Verification items for the finished model (mm, model axes). Face numbers are marked on the shaded views. A direction names the side the tool comes from. Give positions to 0.01 mm unless a question says otherwise; leave off trailing zeros. Write each loop counter-clockwise with the first axis right and the second up, starting at its lowest first coordinate (ties: lowest second). Pieces come first, ordered by that corner, then holes. Notation, with made-up numbers: (73, 13) -> (84, 13) arc R12 cw to (84, 23) -> close; hole circle Ø3 at (12, 29). An arc over 180 degrees is marked (long way). Use one line per item in the form item = value. Start each with the question number.
(1) Set-up check for the marked faces 1 and 2: record each of +Z, -Z, +X, -X, +Y, -Y from which the full face is reachable in a straight line by a thin tool's end or side.
(2) Section check D-D, the plane x = 39.5. Record the cut outline in (y, z).
(3) Scan lines: L1, parallel to X at y = 3.9, z = 0; L2, parallel to Z at x = -62.5, y = 6; L3, parallel to Z at x = 22, y = 15. Record each from-to range of solid material in increasing order.
(4) Section check B-B, the plane x = -38.5. Record the cut outline in (y, z), plus the area to 3 significant figures.
(5) Release check for a two-part mould opening along Z. For the marked faces 3, 4, 5 and 6 record: pulls with the +Z half, pulls with the -Z half, needs draft (parallel to the pull), parting line crosses it, or undercut.
(6) Depth check by flat-ended pin: pin 1 Ø5 at (x, z) = (-31, 19.5) entering from +Y; pin 2 Ø8 at (x, z) = (39.5, -0.5) entering from +Y; pin 3 Ø10 at (y, z) = (13.5, 6.5) entering from -X. Enter the tip coordinate at first touch or a pass-through.
(7) Section check A-A, the plane y = 5. Record the cut outline in (x, z) (3 decimals).
(8) Section check C-C, the plane x = 55. Record the cut outline in (y, z), plus the area to 3 significant figures.
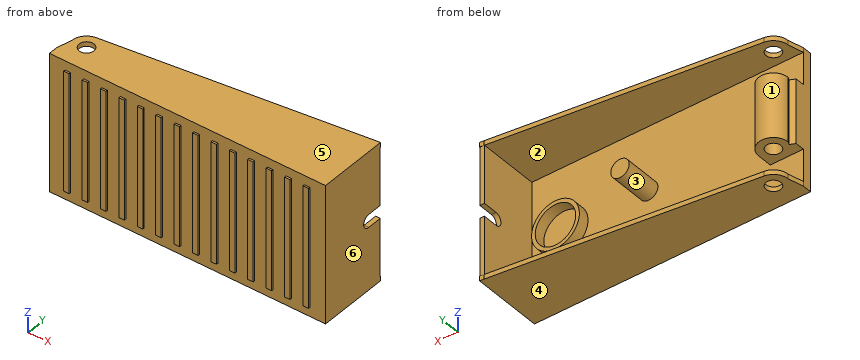
from build123d import *

# Parameters (mm, degrees)
SKETCH2_W               = 150
SKETCH2_H               = 75
BOSS_EXTRUDE1_DEPTH     = 2.5
SKETCH3_R               = 4
BOSS_EXTRUDE2_DEPTH     = 17.5
SKETCH4_R               = 5
BOSS_EXTRUDE3_DEPTH     = 20
SKETCH7_R               = 13
SKETCH7_R_2             = 11
BOSS_EXTRUDE4_DEPTH     = 6
BOSS_EXTRUDE5_START     = 37.5
BOSS_EXTRUDE5_DEPTH     = 2.5
BOSS_EXTRUDE6_START     = -35
BOSS_EXTRUDE6_DEPTH     = 2.5
BOSS_EXTRUDE7_DEPTH     = 2.5
SKETCH11_W              = 3
SKETCH11_H              = 65
BOSS_EXTRUDE8_DEPTH     = 1
CUT_EXTRUDE1_DEPTH      = 112.930169188
CUT_EXTRUDE1_DEPTH_BACK = 112.930169188
SKETCH12_R              = 4


with BuildPart() as part:
    # Sketch2 → Boss-Extrude1 (new, symmetric)
    with BuildSketch(Plane(origin=(0, 0, 0), x_dir=(1, 0, 0), z_dir=(0, 1, 0))):
        Rectangle(SKETCH2_W, SKETCH2_H)
    extrude(amount=BOSS_EXTRUDE1_DEPTH, both=True)

    # Sketch3 → Boss-Extrude2 (add, symmetric)
    with BuildSketch(Plane.XY):
        with BuildLine():
            Line((-57, 10.5), (-57, 2.5))
            Line((-57, 2.5), (-75, 2.5))
            Line((-75, 2.5), (-75, 7.5))
            Line((-75, 7.5), (-72.208145726, 8.801863029))
            Line((-72.208145726, 8.801863029), (-73, 10.5))
            ThreePointArc((-73, 10.5), (-65, 18.5), (-57, 10.5))
        make_face()
        with Locations((-65, 10.5)):
            Circle(SKETCH3_R, mode=Mode.SUBTRACT)
    extrude(amount=BOSS_EXTRUDE2_DEPTH, both=True)

    # Sketch4 → Boss-Extrude3 (add)
    with BuildSketch(Plane(origin=(0, 2.5, 0), x_dir=(1, 0, 0), z_dir=(0, 1, 0))):
        with Locations(Location((9, 0, 0), (0, 0, 270))):
            Circle(SKETCH4_R)
    extrude(amount=BOSS_EXTRUDE3_DEPTH)

    # Sketch7 → Boss-Extrude4 (add)
    with BuildSketch(Plane(origin=(0, 2.5, 0), x_dir=(1, 0, 0), z_dir=(0, 1, 0))):
        with Locations(Location((55, 0, 0), (0, 0, 270))):
            Circle(SKETCH7_R)
        with Locations(Location((55, 0, 0), (0, 0, 270))):
            Circle(SKETCH7_R_2, mode=Mode.SUBTRACT)
    extrude(amount=BOSS_EXTRUDE4_DEPTH)

    # Sketch9 → Boss-Extrude5 (add)
    with BuildSketch(Plane.XY.offset(BOSS_EXTRUDE5_START)):
        with BuildLine():
            Line((75, 35.754199396), (75, 2.5))
            Line((75, 2.5), (-75, 2.5))
            Line((-75, 2.5), (-73, 10.5))
            ThreePointArc((-73, 10.5), (-70.991725081, 15.800870736), (-65.975192361, 18.440340034))
            Line((-65.975192361, 18.440340034), (75, 35.754199396))
        make_face()
    extrude(amount=-BOSS_EXTRUDE5_DEPTH)

    # Sketch9<2> → Boss-Extrude6 (add)
    with BuildSketch(Plane.XY.offset(BOSS_EXTRUDE6_START)):
        with BuildLine():
            Line((75, 35.754199396), (75, 2.5))
            Line((75, 2.5), (-75, 2.5))
            Line((-75, 2.5), (-73, 10.5))
            ThreePointArc((-73, 10.5), (-70.991725081, 15.800870736), (-65.975192361, 18.440340034))
            Line((-65.975192361, 18.440340034), (75, 35.754199396))
        make_face()
    extrude(amount=-BOSS_EXTRUDE6_DEPTH)

    # Sketch10 → Boss-Extrude7 (add)
    with BuildSketch(Plane(origin=(75, 0, 0), x_dir=(0, 0, -1), z_dir=(1, 0, 0))):
        with BuildLine():
            Line((37.5, 35.5), (37.5, -2.5))
            Line((37.5, -2.5), (-37.5, -2.5))
            Line((-37.5, -2.5), (-37.5, 35.5))
            Line((-37.5, 35.5), (-3.5, 35.5))
            Line((-3.5, 35.5), (-3.5, 27.5))
            ThreePointArc((-3.5, 27.5), (0, 24), (3.5, 27.5))
            Line((3.5, 27.5), (3.5, 35.5))
            Line((3.5, 35.5), (37.5, 35.5))
        make_face()
    extrude(amount=-BOSS_EXTRUDE7_DEPTH)

    # Sketch11 → Boss-Extrude8 (add)
    with BuildSketch(Plane.XZ.offset(2.5)):
        with Locations((-45, 0)):
            Rectangle(SKETCH11_W, SKETCH11_H)
        with Locations((-35, 0)):
            Rectangle(SKETCH11_W, SKETCH11_H)
        with Locations((-25, 0)):
            Rectangle(SKETCH11_W, SKETCH11_H)
        with Locations((-15, 0)):
            Rectangle(SKETCH11_W, SKETCH11_H)
        with Locations((-5, 0)):
            Rectangle(SKETCH11_W, SKETCH11_H)
        with Locations((5, 0)):
            Rectangle(SKETCH11_W, SKETCH11_H)
        with Locations((15, 0)):
            Rectangle(SKETCH11_W, SKETCH11_H)
        with Locations((25, 0)):
            Rectangle(SKETCH11_W, SKETCH11_H)
        with Locations((35, 0)):
            Rectangle(SKETCH11_W, SKETCH11_H)
        with Locations((45, 0)):
            Rectangle(SKETCH11_W, SKETCH11_H)
        with Locations((55, 0)):
            Rectangle(SKETCH11_W, SKETCH11_H)
        with Locations((65, 0)):
            Rectangle(SKETCH11_W, SKETCH11_H)
        with Locations((-65, 0)):
            Rectangle(SKETCH11_W, SKETCH11_H)
        with Locations((-55, 0)):
            Rectangle(SKETCH11_W, SKETCH11_H)
    extrude(amount=BOSS_EXTRUDE8_DEPTH)

    # Sketch12 → Cut-Extrude1 (cut, two sides: drawn at the far end of the back side and taken through both)
    with BuildSketch(Plane(origin=(0, 0, -37.5), x_dir=(-1, 0, 0), z_dir=(0, 0, -1)).offset(-CUT_EXTRUDE1_DEPTH_BACK)):
        with Locations(Location((65, 10.5, 0), (0, 0, 180))):
            Circle(SKETCH12_R)
    extrude(amount=CUT_EXTRUDE1_DEPTH + CUT_EXTRUDE1_DEPTH_BACK, mode=Mode.SUBTRACT)


solid = part.part
Completed:
q1.face_1 = +Y
q1.face_2 = -X, +Y
q2.outline = (-2.5, -37.5) -> (31.39, -37.5) -> (31.39, -35) -> (2.5, -35) -> (2.5, 35) -> (31.39, 35) -> (31.39, 37.5) -> (-2.5, 37.5) -> close
q3.L1 = -75 to -57, 4 to 14, 42 to 44, 66 to 68, 72.5 to 75
q3.L2 = -37.5 to -35, -17.5 to 17.5, 35 to 37.5
q3.L3 = -37.5 to -35, 35 to 37.5
q4.outline = (-2.5, -37.5) -> (21.81, -37.5) -> (21.81, -35) -> (2.5, -35) -> (2.5, 35) -> (21.81, 35) -> (21.81, 37.5) -> (-2.5, 37.5) -> close
q4.area = 472 mm²
q5.face_3 = undercut
q5.face_4 = pulls with the -Z half
q5.face_5 = pulls with the +Z half
q5.face_6 = needs draft
q6.pin_1 = 2.5
q6.pin_2 = 8.5
q6.pin_3 = -73
q7.outline = (-75, -17.5) -> (-57, -17.5) -> (-57, 17.5) -> (-75, 17.5) -> close; (-74.375, -37.5) -> (75, -37.5) -> (75, 37.5) -> (-74.375, 37.5) -> (-74.375, 35) -> (72.5, 35) -> (72.5, -35) -> (-74.375, -35) -> close; circle Ø10 at (9, 0); circle Ø26 at (55, 0); hole circle Ø22 at (55, 0)
q8.outline = (-3.5, -32.5) -> (-2.5, -32.5) -> (-2.5, -37.5) -> (33.3, -37.5) -> (33.3, -35) -> (2.5, -35) -> (2.5, -13) -> (8.5, -13) -> (8.5, -11) -> (2.5, -11) -> (2.5, 11) -> (8.5, 11) -> (8.5, 13) -> (2.5, 13) -> (2.5, 35) -> (33.3, 35) -> (33.3, 37.5) -> (-2.5, 37.5) -> (-2.5, 32.5) -> (-3.5, 32.5) -> close
q8.area = 618 mm²
